```python
from build123d import *

# Parameters (mm, degrees)
SKETCH_1_W           = 48.51
SKETCH_1_H           = 34
SKETCH_1_W_2         = 28.51
SKETCH_1_H_2         = 14
EXTRUDE_1_DEPTH      = 12.25
SKETCH_2_R           = 1.91
CUT_EXTRUDE_1_DEPTH  = 33.05257439
SKETCH_4_W           = 13
SKETCH_4_H           = 13.91
EXTRUDE_1_2_DEPTH    = 74.82
SKETCH_5_W           = 13.91
SKETCH_5_H           = 16.23
EXTRUDE_2_DEPTH      = 23.57
SKETCH_7_R           = 24.5
SKETCH_7_R_2         = 14.5
EXTRUDE_2_2_DEPTH    = 16.23
EXTRUDE_3_DEPTH      = 13.15
EXTRUDE_3_DEPTH_BACK = 7
SKETCH_9_W           = 13.91
SKETCH_9_H           = 16.23


with BuildPart() as part:
    # 草圖1 → Extrude 1 (new body)
    with BuildSketch(Plane(origin=(0, 0, 0), x_dir=(1, 0, 0), z_dir=(0, 1, 0))):
        Rectangle(SKETCH_1_W, SKETCH_1_H)
        Rectangle(SKETCH_1_W_2, SKETCH_1_H_2, mode=Mode.SUBTRACT)
    extrude(amount=EXTRUDE_1_DEPTH)

    # 草圖2 → 除料-伸長1 (cut, through all)
    with BuildSketch(Plane(origin=(0, 12.25, 0), x_dir=(1, 0, 0), z_dir=(0, 1, 0))):
        with Locations(Location((-19.255, 0, 0), (0, 0, 270))):
            Circle(SKETCH_2_R)
        with Locations(Location((19.255, 0, 0), (0, 0, 270))):
            Circle(SKETCH_2_R)
    extrude(amount=-CUT_EXTRUDE_1_DEPTH, mode=Mode.SUBTRACT)

    # 草圖4 → Extrude 1 2 (add)
    with BuildSketch(Plane.XZ):
        with Locations((17.755, 0)):
            Rectangle(SKETCH_4_W, SKETCH_4_H)
    extrude(amount=EXTRUDE_1_2_DEPTH)

    # 草圖5 → Extrude 2 (add)
    with BuildSketch(Plane.ZY.offset(-11.255)):
        with Locations((0, -66.705)):
            Rectangle(SKETCH_5_W, SKETCH_5_H)
    extrude(amount=EXTRUDE_2_DEPTH)

    # 草圖7 → Extrude 2 2 (add)
    with BuildSketch(Plane.XZ.offset(74.82)):
        with Locations((-30.978154344, 0)):
            Circle(SKETCH_7_R)
        with Locations((-30.978154344, 0)):
            Circle(SKETCH_7_R_2, mode=Mode.SUBTRACT)
    extrude(amount=-EXTRUDE_2_2_DEPTH)

    # 草圖9 → 填料-伸長3 (add, two sides: drawn at the far end of the back side and taken through both)
    with BuildSketch(Plane(origin=(-60, 0, 0), x_dir=(0, 0, -1), z_dir=(1, 0, 0)).offset(-EXTRUDE_3_DEPTH_BACK)):
        with Locations((0, -66.705)):
            Rectangle(SKETCH_9_W, SKETCH_9_H)
    extrude(amount=EXTRUDE_3_DEPTH + EXTRUDE_3_DEPTH_BACK)


solid = part.part
```
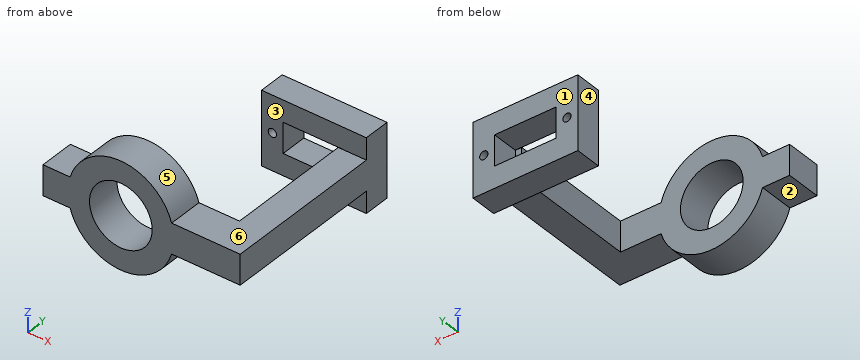
Design review of the part built by this model. Coordinates are the model's own, in mm. Face numbers are marked on the shaded views. A direction names the side the tool comes from. Coordinates: 2 decimals unless noted, no trailing zeros. Order: outer loops, then holes, each group sorted by start corner. A loop starts at its lowest first (then second) coordinate and runs counter-clockwise, first axis right, second up.
1) Take a section at C-C, the plane z = -10.5. Give the boundary of the cut face in (x, y) (3 decimals), and give its area (3 significant figures).
2) Wall thickness on line 1 along X through (y, z) = (5.5, 0) (3 decimals); line 2 along Y through (x, z) = (-51, 4); line 3 along X through (y, z) = (-4.5, -4.5) (3 decimals): over which ranges is each line inside the solid? List them lowest first.
3) Take a section at A-A, the plane z = 0. Give the boundary of the cut face in (x, y) (3 decimals), and give its area (3 significant figures).
4) For the marked faces 4, 5 and 6, list the 3-axis set-ups (+Z, -Z, +X, -X, +Y, -Y) from which the entire face can be reached by the end or side of a thin tool; tool diameter is ignored.
5) Mouldability with a two-part tool opening along Y and no side actions: class the marked faces 1, 2 and 3 as +Y half, -Y half, draft (parallel to the pull), parting line (faces both ways), or undercut.
6) Clearance check with flat-ended pins moving along their axes: pin 1 (6 mm diameter, centred on x = 10.5, y = 4, fed in from -Z); pin 2 (11 mm diameter, centred on y = -22, z = 1.5, fed in from -X) (3 decimals); pin 3 (4 mm diameter, centred on x = -63, y = -64, fed in from -Z) (3 decimals); pin 4 (6 mm diameter, centred on x = 19.255, z = 0, fed in from +Y). State where each tip first meets the part, or that it passes through.
7) Take a section at B-B, the plane x = -2.5. Give the boundary of the cut face in (y, z) (3 decimals), and give its area (3 significant figures).
8) Take a section at D-D, the plane x = -37. Give the boundary of the cut face in (y, z).
Returned:
1. outline: (-53.114, -74.82) - (-40.978, -74.82) - (-40.978, -58.59) - (-53.114, -58.59) - close; (-24.255, 0) - (24.255, 0) - (24.255, 12.25) - (-24.255, 12.25) - close; (-20.978, -74.82) - (-8.842, -74.82) - (-8.842, -58.59) - (-20.978, -58.59) - close
1. area: 988 mm2
2. line 1: x = -24.255 to -21.165, -17.345 to -14.255, 14.255 to 17.345, 21.165 to 24.255
2. line 2: y = -74.82 to -58.59
2. line 3: x = 11.255 to 24.255
3. outline: (-67, -74.82) - (-45.478, -74.82) - (-45.478, -58.59) - (-67, -58.59) - close; (-24.255, 0) - (-21.165, 0) - (-21.165, 12.25) - (-24.255, 12.25) - close; (-17.345, 0) - (-14.255, 0) - (-14.255, 12.25) - (-17.345, 12.25) - close; (-16.478, -74.82) - (24.255, -74.82) - (24.255, 12.25) - (21.165, 12.25) - (21.165, 0) - (17.345, 0) - (17.345, 12.25) - (14.255, 12.25) - (14.255, 0) - (11.255, 0) - (11.255, -58.59) - (-16.478, -58.59) - close
3. area: 1,920 mm2
4. face 4: +Z, -Z, -X, +Y
4. face 5: +Z, -Y
4. face 6: +Z, +X, -Y
5. face 1: +Y half
5. face 2: draft
5. face 3: undercut
6. pin 1: stops at z = -17
6. pin 2: stops at x = 11.255
6. pin 3: stops at z = -6.955
6. pin 4: stops at y = 12.25
7. outline: (-74.82, -6.955) - (-58.59, -6.955) - (-58.59, 6.955) - (-74.82, 6.955) - close; (0, -17) - (12.25, -17) - (12.25, -7) - (0, -7) - close; (0, 7) - (12.25, 7) - (12.25, 17) - (0, 17) - close
7. area: 471 mm2
8. outline: (-74.82, -23.75) - (-58.59, -23.75) - (-58.59, -13.19) - (-74.82, -13.19) - close; (-74.82, 13.19) - (-58.59, 13.19) - (-58.59, 23.75) - (-74.82, 23.75) - close
